```python
from build123d import *

# Parameters (mm, degrees)
F0_W     = 32.155059278
F0_H     = 22.1614539623
F1_DEPTH = 91.5020089597
F2_SIZE  = 12.7


with BuildPart() as f1:
    # F0 (on Top) → F1 (new body)
    with BuildSketch(Plane.XY):
        Polygon((0, 28.1687378883), (0, 50.3301918507), (32.155059278, 50.3301918507), (32.155059278, 111.7442771792), (-89.617818594, 111.7442771792), (-89.617818594, 28.1687378883), align=None)
        with Locations((16.077529639, 39.2494648695)):
            Rectangle(F0_W, F0_H)
        Polygon((65.0401264429, 50.3301918507), (32.155059278, 50.3301918507), (32.155059278, 28.1687378883), (0, 28.1687378883), (0, 0), (65.0401264429, 0), align=None)
    extrude(amount=F1_DEPTH)

    # F2
    f2_edges = [f1.edges().sort_by_distance(p)[0] for p in [
        (-44.808909, 28.168738, 91.502009),
        (0, 14.084369, 91.502009),
        (32.520063, 0, 91.502009),
        (65.040126, 25.165096, 91.502009),
        (48.597593, 50.330192, 91.502009),
        (32.155059, 81.037235, 91.502009),
    ]]
    chamfer(f2_edges, length=F2_SIZE)


solid = f1.part
```
The listing builds one solid part. Answer for the finished solid, in the listing's coordinates (mm). A direction names the side the tool comes from. Coordinates: 2 decimals unless noted, no trailing zeros. Write each loop counter-clockwise with the first axis right and the second up, starting at its lowest first coordinate (ties: lowest second). Pieces come first, ordered by that corner, then holes. Notation, with made-up numbers: M -29,51 L -24,51 A26 cw -24,71 Z; hole C 37,58.25 d9. An arc over 180 degrees is marked long. Use a Markdown table: item, result. Add a question column.
1. Section C-C (y = 45.5) is taken. Give the vertices of the cut face in (x, z), plus the area to 3 significant figures.
2. Section D-D (y = 99) is taken. Give the vertices of the cut face in (x, z), plus the area to 3 significant figures.
3. Which of the six approach directions +Z, -Z, +X, -X, +Y, -Y give full straight-line access (tool end or side, diameter ignored) to faces 1 (the flat face through (32, 0, 39)), 2 (the flat face through (32.155, 81, 39)), 3 (the flat face through (-45, 28.169, 39)), 4 (the flat face through (6.4, 20.7, 85.2)), 5 (the flat face through (42.57, 43.89, 85.24))?
4. Section B-B (z = 28.5) is taken. Give the vertices of the cut face in (x, y).
5. Section A-A (x = -18.5) is taken. Give the vertices of the cut face in (y, z).
6. Given P1, Ø10, axis at x = 22, y = 62.5, coming from the -Z side; P2, Ø1.5, axis at x = -8, y = 40, coming from the +Z side; P3, Ø8.5, axis at y = 20, z = 50.5, coming from the -X side; P4, Ø6, axis at x = -57.5, y = 22.5, coming from the +Z side, each flat-ended and moving along its own axis, determine where each tip first touches the part or whether it passes through.
7. Straight lines are drawn through the part: line 1 along X through (y, z) = (68, 5.5); line 2 along Y through (x, z) = (52, 55); line 3 along Y through (x, z) = (-50, 62). For each, find the intervals that lie inside material, in ascending order. Write a range as [from, to].
Data:
| question | item | result |
|---|---|---|
| 1 | outline | M -89.62,0 L 65.04,0 L 65.04,78.8 L 60.21,83.63 L 27.32,83.63 L 19.46,91.5 L -89.62,91.5 Z |
| 1 | area | 13,800 mm2 |
| 2 | outline | M -89.62,0 L 32.16,0 L 32.16,78.8 L 19.46,91.5 L -89.62,91.5 Z |
| 2 | area | 11,100 mm2 |
| 3 | face 1 | +Z, -Z, +X, -X, -Y |
| 3 | face 2 | +Z, -Z, +X, +Y |
| 3 | face 3 | +Z, -Z, -X, -Y |
| 3 | face 4 | +Z, -X, -Y |
| 3 | face 5 | +Z, +X, +Y |
| 4 | outline | M -89.62,28.17 L 0,28.17 L 0,0 L 65.04,0 L 65.04,50.33 L 32.16,50.33 L 32.16,111.74 L -89.62,111.74 Z |
| 5 | outline | M 28.17,0 L 111.74,0 L 111.74,91.5 L 40.87,91.5 L 28.17,78.8 Z |
| 6 | P1 | stops at z = 0 |
| 6 | P2 | stops at z = 91.38 |
| 6 | P3 | stops at x = 0 |
| 6 | P4 | passes through |
| 7 | line 1 | x = [-89.62, 32.16] |
| 7 | line 2 | y = [0, 50.33] |
| 7 | line 3 | y = [28.17, 111.74] |
